Autodesk Inventor part; units mm, degrees
ref_plane "YZ Plane" through (0, 0, 0) normal (1, 0, 0) x (0, 1, 0)
ref_plane "XZ Plane" through (0, 0, 0) normal (0, 1, 0) x (-1, 0, 0)
ref_plane "XY Plane" through (0, 0, 0) normal (0, 0, 1) x (1, 0, 0)
sketch "Sketch1" plane through (0, 0, 0) normal (0, 1, 0) x (-1, 0, 0)
  line L0 (-30, 25) -> (30, 25)
  line L1 (30, 25) -> (30, -25)
  line L2 (30, -25) -> (-30, -25)
  line L3 (-30, -25) -> (-30, 25)
  line L4 (-30, 25) -> (30, -25) construction
  line L5 (30, 25) -> (-30, -25) construction
  point P0 (0, 0)
  dimension "d0" = 60
  dimension "d1" = 50
extrude "Extrusion1" add sketch "Sketch1" along normal blind 4
sketch "Sketch2" plane through (0, 4, 0) normal (0, 1, 0) x (1, 0, 0)
  line L0 (24.55, -16.5) -> (-24.55, -16.5)
  line L1 (-24.55, -16.5) -> (-24.55, 16.5)
  line L2 (-24.55, 16.5) -> (24.55, 16.5)
  line L3 (24.55, 16.5) -> (24.55, -16.5)
  line L4 (24.55, -16.5) -> (-24.55, 16.5) construction
  line L5 (-24.55, -16.5) -> (24.55, 16.5) construction
  line L6 (-24.55, 0) -> (-19.05, 0) construction
  arc A0 (-19.05, -5.5) -> (-19.05, 5.5) centre (-19.05, 0) ccw
  circle A1 centre (-19.05, 0) radius 1.5
  line L7 (-24.55, -5.5) -> (-19.05, -5.5)
  line L8 (-19.05, 5.5) -> (-24.55, 5.5)
  line L9 (0, 0) -> (0, 7.8655) construction
  arc A2 (19.05, 5.5) -> (19.05, -5.5) centre (19.05, 0) ccw
  circle A3 centre (19.05, 0) radius 1.5
  line L10 (24.55, -5.5) -> (19.05, -5.5)
  line L11 (19.05, 5.5) -> (24.55, 5.5)
  point P0 (0, 0)
  dimension "d4" = 49.1
  dimension "d5" = 33
  dimension "d6" = 5.5
  dimension "d7" = 3
extrude "Extrusion2" cut sketch "Sketch2" against normal through all contours L0 L1 L7 A0 L8 L2 L3 L11 A2 L10 | A1 | A3
sketch "Sketch3" plane through (0, 0, 0) normal (0, -1, 0) x (1, 0, 0)
  line L0 (-30, 25) -> (30, 25)
  line L1 (-30, 25) -> (-34, 25)
  line L2 (-34, 25) -> (-34, 5)
  line L3 (-34, 5) -> (-30, 5)
  line L4 (-30, 5) -> (-30, 25)
  line L5 (-34, 25) -> (-10, 25)
  line L6 (-10, 25) -> (-10, 29)
  line L7 (-10, 29) -> (-34, 29)
  line L8 (-34, 29) -> (-34, 25)
  line L9 (-30, -25) -> (-30, 25)
  line L10 (-30, 0) -> (-43.5069, 0) construction
  line L11 (-30, -25) -> (-34, -25)
  line L12 (-34, -25) -> (-34, -5)
  line L13 (-34, -5) -> (-30, -5)
  line L14 (-30, -5) -> (-30, -25)
  line L15 (-34, -25) -> (-10, -25)
  line L16 (-10, -25) -> (-10, -29)
  line L17 (-10, -29) -> (-34, -29)
  line L18 (-34, -29) -> (-34, -25)
  line L19 (0, 25) -> (0, 63.1817) construction
  line L20 (30, 25) -> (34, 25)
  line L21 (34, 25) -> (34, 5)
  line L22 (34, 5) -> (30, 5)
  line L23 (30, 5) -> (30, 25)
  line L24 (34, 25) -> (10, 25)
  line L25 (10, 25) -> (10, 29)
  line L26 (10, 29) -> (34, 29)
  line L27 (34, 29) -> (34, 25)
  line L28 (30, -25) -> (30, 25)
  line L29 (30, 0) -> (43.5069, 0) construction
  line L30 (30, -25) -> (34, -25)
  line L31 (34, -25) -> (34, -5)
  line L32 (34, -5) -> (30, -5)
  line L33 (30, -5) -> (30, -25)
  line L34 (34, -25) -> (10, -25)
  line L35 (10, -25) -> (10, -29)
  line L36 (10, -29) -> (34, -29)
  line L37 (34, -29) -> (34, -25)
  line L38 (30, -25) -> (30, -29)
  line L39 (30, 25) -> (30, 29)
  point P0 (0, 0)
  point P1 (-30, -25)
  point P2 (-30, -5)
  point P3 (30, -5)
  point P4 (30, -25)
  point P5 (30, -25)
  dimension "d21" = 4
  dimension "d22" = 20
  dimension "d23" = 24
  dimension "d24" = 4
extrude "Extrusion3" add sketch "Sketch3" along normal blind 15 and the other way blind 4 contours L20 L21 L22 L23 | L11 L12 L13 L9
fillet "Fillet1" radius 3 12 edges at (24.55, 2, -16.5) (24.55, 2, -5.5) (24.55, 2, 16.5) (24.55, 2, 5.5) (-24.55, 2, -16.5) (-24.55, 2, -5.5) (-24.55, 2, 5.5) (-24.55, 2, 16.5) (19.05, 2, 5.5) (19.05, 2, -5.5) (-19.05, 2, -5.5) (-19.05, 2, 5.5)
sketch "Sketch7" plane through (-30, 0, -5) normal (1, 0, 0) x (0, 0, -1)
  line L0 (0, -15) -> (20, -15)
  line L1 (10, -15) -> (10, 0)
  line L2 (20, 0) -> (0, 0)
  circle A0 centre (10, -7.5) radius 1.5
  line L3 (-5, 0) -> (-5, -12.3055)
  circle A1 centre (-20, -7.5) radius 1.5
  dimension "d47" = 3
extrude "Extrusion8" cut sketch "Sketch7" along normal through all both and the other way through all
sketch "Sketch9" plane through (0, -15, 0) normal (0, -1, 0) x (1, 0, 0)
  line L0 (-34, -5) -> (-34, -25)
  line L1 (-30, -25) -> (-30, -5)
  line L2 (-30, -5) -> (-34, -5)
  line L3 (-34, -25) -> (-30, -25)
  line L4 (-34, 5) -> (-30, 5)
  line L5 (-30, 5) -> (-30, 25)
  line L6 (-30, 25) -> (-34, 25)
  line L7 (-34, 25) -> (-34, 5)
  line L8 (30, 29) -> (10, 29)
  line L9 (10, 29) -> (10, 25)
  line L10 (10, 25) -> (30, 25)
  line L11 (30, 25) -> (30, 29)
  line L12 (10, -29) -> (30, -29)
  line L13 (30, -29) -> (30, -25)
  line L14 (30, -25) -> (10, -25)
  line L15 (10, -25) -> (10, -29)
  point P0 (0, 0)
extrude "Extrusion10" cut sketch "Sketch9" against normal blind 3
fillet "Fillet2" radius 10 4 edges at (-32, -12, -5) (-32, -12, -25) (32, -15, 5) (32, -15, 25)
properties part number "LED_mount" material "ABS Plastic"
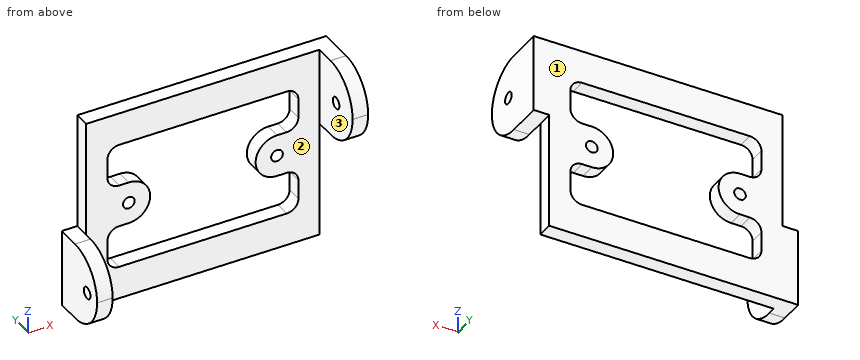
Part model, mm, in its own coordinate system. Face numbers are marked on the shaded views. A direction names the side the tool comes from. Coordinates: 2 decimals unless noted, no trailing zeros. Order: outer loops, then holes, each group sorted by start corner. A loop starts at its lowest first (then second) coordinate and runs counter-clockwise, first axis right, second up. Notation, with made-up numbers: (84.25, -14.75) - (96.25, -14.75) arc R18 ccw to (96.25, 3.25) - close; hole circle Ø4 at (-19.5, 54.25). An arc over 180 degrees is marked (long way). Return JSON: item names as keys, results as strings. Group by question number.
Item 1: Cut at D-D (z = -18.5). List the corners of the cut face in (x, y), plus the area to 3 significant figures.
Item 2: Cut at B-B (x = -15). List the corners of the cut face in (y, z), plus the area to 3 significant figures.
Item 3: Pin check, flat tips, straight feed: pin 1 (1.2 mm diameter, centred on x = -32, y = 0, fed in from +Z); pin 2 (6 mm diameter, centred on x = -25.5, z = 15.5, fed in from -Y); pin 3 (2 mm diameter, centred on y = 1, z = 8.5, fed in from -X). Stop position of each tip, or through.
Item 4: Cut at C-C (y = -7.5). List the corners of the cut face in (x, z), plus the area to 3 significant figures.
Item 5: Drill centre lines: probe 1 along X at (y, z) = (1.45, 0); probe 2 along Y at (x, z) = (31.65, 15); probe 3 along Z at (x, y) = (-21.5, 2.25). Where is each one in solid material? Low to high. Write a range as from..to.
Item 6: Cut at A-A (y = -0.75). List the corners of the cut face in (x, z), plus the area to 3 significant figures.
Item 7: Which spindle directions (+Z, -Z, +X, -X, +Y, -Y) get a long thin tool onto all of the face, cutting with end or side? Do the marked faces 1, 2 and 3. Say none if no direction does.
Check values:
{
 "1": {"outline": "(-34, -11.37) - (-30, -11.37) - (-30, 0) - (30, 0) - (30, 4) - (-34, 4) - close", "area": "301 mm2"},
 "2": {"outline": "(0, -25) - (4, -25) - (4, -16.5) - (0, -16.5) - close; (0, -3.72) - (4, -3.72) - (4, 3.72) - (0, 3.72) - close; (0, 16.5) - (4, 16.5) - (4, 25) - (0, 25) - close", "area": "97.8 mm2"},
 "3": {"pin 1": "stops at z = -5", "pin 2": "stops at y = 0", "pin 3": "stops at x = -30"},
 "4": {"outline": "(-34, -23.35) - (-30, -23.35) - (-30, -16.5) - (-34, -16.5) - close; (-34, -13.5) - (-30, -13.5) - (-30, -6.65) - (-34, -6.65) - close; (30, 5.32) - (34, 5.32) - (34, 13.5) - (30, 13.5) - close; (30, 16.5) - (34, 16.5) - (34, 24.68) - (30, 24.68) - close", "area": "120 mm2"},
 "5": {"probe 1": "x = -30..-20.55, -17.55..-13.55, 13.55..17.55, 20.55..30", "probe 2": "y = -15..-9, -6..4", "probe 3": "z = -25..-16.5, -5.5..5.5, 16.5..25"},
 "6": {"outline": "(-34, -25) - (-30, -25) - (-30, -5) - (-34, -5) - close; (30, 5) - (34, 5) - (34, 25) - (30, 25) - close", "area": "160 mm2"},
 "7": {"face 1": "+Z, -Z, +X, -X, +Y", "face 2": "+Z, -Z, -Y", "face 3": "+Z, -Z, -X, -Y"}
}
